from build123d import *

# Parameters (mm, degrees)
EXTRUDE_1_DEPTH     = 118.5
SKETCH_2_W          = 20
SKETCH_2_H          = 180
CUT_REVOLVE_1_ANGLE = 180


with BuildPart() as part:
    # 草图1 → 凸台-拉伸1 (new, symmetric)
    with BuildSketch(Plane.XY):
        with BuildLine():
            Line((-500, 0), (-300, 0))
            Line((-300, 0), (-300, 80))
            ThreePointArc((-300, 80), (-270, 110), (-240, 80))
            Line((-240, 80), (-240, 0))
            Line((-240, 0), (-60, 0))
            Line((-60, 0), (-60, 120))
            ThreePointArc((-60, 120), (0, 180), (60, 120))
            Line((60, 120), (60, 0))
            Line((60, 0), (240, 0))
            Line((240, 0), (240, 80))
            ThreePointArc((240, 80), (270, 110), (300, 80))
            Line((300, 80), (300, 0))
            Line((300, 0), (500, 0))
            ThreePointArc((500, 0), (0, 500), (-500, 0))
        make_face()
    extrude(amount=EXTRUDE_1_DEPTH, both=True)

    # 草图2 → 切除-旋转1 (revolve, cut)
    with BuildSketch(Plane(origin=(0, 0, 0), x_dir=(1, 0, 0), z_dir=(0, 1, 0))):
        with Locations((500, 0)):
            Rectangle(SKETCH_2_W, SKETCH_2_H)
    revolve(axis=Axis((0, 0, -254.401615848), (0, 0, 1)), revolution_arc=CUT_REVOLVE_1_ANGLE, mode=Mode.SUBTRACT)


solid = part.part
Work out the finished part from the listing and answer in its coordinate system (mm). A direction names the side the tool comes from. Round coordinates to 2 decimals unless told otherwise and drop trailing zeros. Write each loop counter-clockwise with the first axis right and the second up, starting at its lowest first coordinate (ties: lowest second). Pieces come first, ordered by that corner, then holes. Notation, with made-up numbers: M 7,57.5 L 64,57.5 A7 cw 64,68.5 Z; hole C -0.75,70.25 d5. An arc over 180 degrees is marked long. Use a Markdown table: item, result.
1) Which of the six approach directions +Z, -Z, +X, -X, +Y, -Y give full straight-line access (tool end or side, diameter ignored) to faces 4 (the face through (10.77, 489.88, -1.26)), 5 (the face through (-240, 41, 2)), 6 (the face through (-7, 198, 118.5))?
Taken from the geometry:
| item | result |
|---|---|
| face 4 | +Y |
| face 5 | +Z, -Z, -Y |
| face 6 | +Z, +X, -X, +Y, -Y |
2) The part is cut by section A-A on z = -79. Give the vertices of the cut face in (x, y), plus the area to 3 significant figures.
Taken from the geometry:
| item | result |
|---|---|
| outline | M -490,0 L -300,0 L -300,80 A30 cw -240,80 L -240,0 L -60,0 L -60,120 A60 cw 60,120 L 60,0 L 240,0 L 240,80 A30 cw 300,80 L 300,0 L 490,0 A490 ccw Z |
| area | 345,000 mm2 |
3) The part is cut by section D-D on y = 218. Give the vertices of the cut face in (x, z).
Taken from the geometry:
| item | result |
|---|---|
| outline | M -449.97,-118.5 L 449.97,-118.5 L 449.97,-90 L 438.83,-90 L 438.83,90 L 449.97,90 L 449.97,118.5 L -449.97,118.5 L -449.97,90 L -438.83,90 L -438.83,-90 L -449.97,-90 Z |
4) Flat-ended cylindrical pins translate along their axes: pin 1 (3 mm diameter, centred on y = 102, z = 47.5, fed in from +X); pin 2 (6 mm diameter, centred on y = 290, z = -74, fed in from +X); pin 3 (6 mm diameter, centred on x = -56, z = -7, fed in from +Y). Find the tip coordinate at first contact, or state that the pin passes through.
Taken from the geometry:
| item | result |
|---|---|
| pin 1 | stops at x = 479.58 |
| pin 2 | stops at x = 397.15 |
| pin 3 | stops at y = 487.13 |
5) The part is cut by section B-B on x = -346. Give the vertices of the cut face in (y, z).
Taken from the geometry:
| item | result |
|---|---|
| outline | M 0,-118.5 L 360.95,-118.5 L 360.95,-90 L 346.96,-90 L 346.96,90 L 360.95,90 L 360.95,118.5 L 0,118.5 Z |
6) The part is cut by section C-C on y = 154.5. Give the vertices of the cut face in (x, z), plus the area to 3 significant figures.
Taken from the geometry:
| item | result |
|---|---|
| outline | M -475.53,-118.5 L -49.09,-118.5 L -49.09,118.5 L -475.53,118.5 L -475.53,90 L -465.01,90 L -465.01,-90 L -475.53,-90 Z; M 49.09,-118.5 L 475.53,-118.5 L 475.53,-90 L 465.01,-90 L 465.01,90 L 475.53,90 L 475.53,118.5 L 49.09,118.5 Z |
| area | 198,000 mm2 |
7) Determine the mould class of faces 1 (the face through (-7, 198, -118.5)), 2 (the face through (2, 492, 90)), 3 (the face through (-151, 0, 2)) for opening direction Z: pulls with the +Z half, pulls with the -Z half, needs draft (parallel to the pull), parting line crosses it, or undercut.
Taken from the geometry:
| item | result |
|---|---|
| face 1 | pulls with the -Z half |
| face 2 | undercut |
| face 3 | needs draft |
8) Consider line 1 (X direction, y = 106, z = -37); line 2 (X direction, y = 36.5, z = 6.5); line 3 (X direction, y = 400, z = 105). Determine where each line is inside the solid, lowest interval first. Write a range as [from, to].
Taken from the geometry:
| item | result |
|---|---|
| line 1 | x = [-478.4, -284.97], [-255.03, -60], [60, 255.03], [284.97, 478.4] |
| line 2 | x = [-488.64, -300], [-240, -60], [60, 240], [300, 488.64] |
| line 3 | x = [-300, 300] |
